Geometry check sheet. Reference: the model listing, model coordinates, mm. A direction names the side the tool comes from. Give positions to 0.01 mm unless a question says otherwise; leave off trailing zeros. Write each loop counter-clockwise with the first axis right and the second up, starting at its lowest first coordinate (ties: lowest second). Pieces come first, ordered by that corner, then holes. Notation, with made-up numbers: (-19, 41.25) -> (31, 41.25) arc R20 ccw to (31, 70.25) -> close; hole circle Ø3 at (24, -4). An arc over 180 degrees is marked (long way). One line per item, written item: value.
from build123d import *

# Parameters (mm, degrees)
SKETCH1_R                    = 16.5
BOSS_EXTRUDE1_DEPTH          = 5
CHAMFER2_SIZE                = 1
CHAMFER2_SIZE2               = 5
SKETCH3_R                    = 13.5
CUT_EXTRUDE1_DEPTH           = 2.8
SKETCH5_W                    = 1
SKETCH5_H                    = 2
REVOLVE4_ANGLE               = 5
REVOLVE4_OTHER_WAY_ANGLE     = 5
SKETCH6_W                    = 1
SKETCH6_H                    = 2
REVOLVE6_ANGLE               = 5
REVOLVE6_OTHER_WAY_ANGLE     = 5
SKETCH9_W                    = 16.5
SKETCH9_H                    = 2.5
CUT_REVOLVE1_ANGLE           = 85
CUT_REVOLVE1_OTHER_WAY_ANGLE = 10


with BuildPart() as part:
    # Sketch1 → Boss-Extrude1 (new body)
    with BuildSketch(Plane(origin=(0, 0, 0), x_dir=(1, 0, 0), z_dir=(0, 1, 0))):
        with Locations(Location((0, 0, 0), (0, 0, 270))):
            Circle(SKETCH1_R)
    extrude(amount=BOSS_EXTRUDE1_DEPTH)

    # Chamfer2
    chamfer2_edges = [part.edges().sort_by_distance(p)[0] for p in [
        (0, 5, -16.5),
    ]]
    chamfer2_side = [part.faces().sort_by_distance(p)[0] for p in [
        (0, 2.5, -16.5),
    ]]
    chamfer(chamfer2_edges, length=CHAMFER2_SIZE, length2=CHAMFER2_SIZE2, reference=chamfer2_side[0])

    # Sketch3 → Cut-Extrude1 (cut)
    with BuildSketch(Plane(origin=(0, 0, 0), x_dir=(1, 0, 0), z_dir=(0, 1, 0))):
        with Locations(Location((0, 0, 0), (0, 0, 270))):
            Circle(SKETCH3_R)
    extrude(amount=CUT_EXTRUDE1_DEPTH, mode=Mode.SUBTRACT)

    # Sketch5 → Revolve4 (revolve)
    with BuildSketch(Plane(origin=(0, 0, 0), x_dir=(0, 0, -1), z_dir=(1, 0, 0))):
        with Locations((17, 1)):
            Rectangle(SKETCH5_W, SKETCH5_H)
    revolve(axis=Axis((0, 0, 0), (0, 1, 0)), revolution_arc=REVOLVE4_ANGLE)

    # Sketch5 → Revolve4 other way (revolve)
    with BuildSketch(Plane(origin=(0, 0, 0), x_dir=(0, 0, -1), z_dir=(1, 0, 0))):
        with Locations((17, 1)):
            Rectangle(SKETCH5_W, SKETCH5_H)
    revolve(axis=Axis((0, 0, 0), (0, -1, 0)), revolution_arc=REVOLVE4_OTHER_WAY_ANGLE)

    # Sketch6 → Revolve6 (revolve)
    with BuildSketch(Plane(origin=(0, 0, 0), x_dir=(0, 0, -1), z_dir=(1, 0, 0))):
        with Locations((-17, 1)):
            Rectangle(SKETCH6_W, SKETCH6_H)
    revolve(axis=Axis((0, 0, 0), (0, 1, 0)), revolution_arc=REVOLVE6_ANGLE)

    # Sketch6 → Revolve6 other way (revolve)
    with BuildSketch(Plane(origin=(0, 0, 0), x_dir=(0, 0, -1), z_dir=(1, 0, 0))):
        with Locations((-17, 1)):
            Rectangle(SKETCH6_W, SKETCH6_H)
    revolve(axis=Axis((0, 0, 0), (0, -1, 0)), revolution_arc=REVOLVE6_OTHER_WAY_ANGLE)

    # Sketch9 → Cut-Revolve1 (revolve, cut)
    with BuildSketch(Plane.XY):
        with Locations((-8.25, 1.25)):
            Rectangle(SKETCH9_W, SKETCH9_H)
    revolve(axis=Axis((0, 0, 0), (0, 1, 0)), revolution_arc=CUT_REVOLVE1_ANGLE, mode=Mode.SUBTRACT)

    # Sketch9 → Cut-Revolve1 other way (revolve, cut)
    with BuildSketch(Plane.XY):
        with Locations((-8.25, 1.25)):
            Rectangle(SKETCH9_W, SKETCH9_H)
    revolve(axis=Axis((0, 0, 0), (0, -1, 0)), revolution_arc=CUT_REVOLVE1_OTHER_WAY_ANGLE, mode=Mode.SUBTRACT)


solid = part.part
1) Depth check by flat-ended pin: pin 1 Ø2 at (x, z) = (-5.5, -3) entering from -Y; pin 2 Ø0.9 at (x, z) = (-0.5, -17) entering from +Y; pin 3 Ø2 at (y, z) = (4, -3.5) entering from -X. Enter the tip coordinate at first touch or a pass-through.
Verdict:
pin 1: y = 2.8
pin 2: y = 2
pin 3: x = -16.31
2) Sectioned sample at C-C on x = 0. Record the cut outline in (y, z).
Verdict:
outline: (0, -17.5) -> (2, -17.5) -> (2, -16.5) -> (4, -16.5) -> (5, -11.5) -> (5, 11.5) -> (4, 16.5) -> (2, 16.5) -> (2, 17.5) -> (0, 17.5) -> (0, 13.5) -> (2.8, 13.5) -> (2.8, -13.5) -> (0, -13.5) -> close
3) Sectioned sample at B-B on z = 0. Record the cut outline in (x, y), plus the area to 3 significant figures.
Verdict:
outline: (-16.5, 2.5) -> (-13.5, 2.5) -> (-13.5, 2.8) -> (13.5, 2.8) -> (13.5, 0) -> (16.5, 0) -> (16.5, 4) -> (11.5, 5) -> (-11.5, 5) -> (-16.5, 4) -> close
area: 76.9 mm^2
4) Tool access check on faces 5 (the flat face through (1.48, 1.01, -16.93)), 6 (the flat face through (-1.48, 1.01, -16.93)), 7 (the flat face through (-14.793, 1.268, -2.608)). Record the directions out of +Z, -Z, +X, -X, +Y, -Y that give a thin tool (end or side, any length) a straight path to the whole face; none if there is none.
Verdict:
face 5: +X, +Y, -Y
face 6: -X, +Y, -Y
face 7: +Z, -X, -Y
5) Scan lines: probe 1 along X at (y, z) = (1.2, -7); probe 2 along X at (y, z) = (1.15, 0); probe 3 along Y at (x, z) = (-5.5, -7). Record each from-to range of solid material in increasing order.
Verdict:
probe 1: -14.94 to -11.54, 11.54 to 14.94
probe 2: 13.5 to 16.5
probe 3: 2.8 to 5
6) Sectioned sample at A-A on y = 1. Record the cut outline in (x, z), plus the area to 3 significant figures.
Verdict:
outline: (-16.25, -2.87) arc R16.5 ccw to (-1.44, -16.44) -> (-1.53, -17.43) arc R17.5 ccw to (1.53, -17.43) -> (1.44, -16.44) arc R16.5 ccw to (1.44, 16.44) -> (1.53, 17.43) arc R17.5 ccw to (-1.53, 17.43) -> (-1.18, 13.45) arc R13.5 cw (long way) to (-13.29, -2.34) -> close
area: 214 mm^2
7) Mould release check, pull along Z, two halves, no side actions. Record for faces 1 (the conical face through (-11.46, 4.95, -2.55)), 2 (the flat face through (-1.353, 1.268, 15.469)), 3 (the flat face through (0, 2.8, 0)), 4 (the cylindrical face through (0, 1, 17.5)): released by +Z, released by -Z, zero draft, split by the parting line, or undercut.
Verdict:
face 1: split by the parting line
face 2: undercut
face 3: undercut
face 4: released by +Z
